Can you work these out from the model? Positions are in its coordinate system, mm. A direction names the side the tool comes from. Coordinates: 2 decimals unless noted, no trailing zeros. Order: outer loops, then holes, each group sorted by start corner. A loop starts at its lowest first (then second) coordinate and runs counter-clockwise, first axis right, second up. Notation, with made-up numbers: (-4.5, 19) -> (0.5, 19) arc R6 ccw to (0.5, 29) -> close; hole circle Ø5 at (45.25, -4.75). An arc over 180 degrees is marked (long way). Answer in a Markdown table with one row per item. Add a question column.
1. Imagine slicing it at C-C on x = 0. State how many separate pieces and enclosed holes the cut face has, plus the area to 3 significant figures.
2. On a 3-axis mill with a long thin cutter (end or side, diameter ignored), from which of +Z, -Z, +X, -X, +Y, -Y can I reach the whole of each face in a straight line? I mean faces 5 (the face through (52.997, 6.958, -0.535)), 6 (the face through (34, 20, 15)), 7 (the face through (15, 2, 22)). Say none if no direction works.
3. Imagine slicing it at B-B on y = 6.25. Write out the boundary of the cut face in (x, z), plus the area to 3 significant figures.
4. If I drill on line 1 along Y through (x, z) = (-16, -44); line 2 along Z through (x, y) = (12, 19); line 3 along X through (y, z) = (9.5, -24), over which ranges is the centre line in solid material (lowest first)? Write a range as [from, to].
5. Imagine slicing it at A-A on y = 19.75. Write out the boundary of the cut face in (x, z).
6. Will these pins go through, and if not, where does the flat tip stop? pin 1 (5 mm diameter, centred on x = 39, y = 11, fed in from +Z); pin 2 (3 mm diameter, centred on x = 1.5, y = 2, fed in from +Z); pin 3 (5 mm diameter, centred on y = 4, z = 29, fed in from +X); pin 4 (1.6 mm diameter, centred on x = 35, y = 20, fed in from +Z).
7. We'd pull the mould along Z, two halves only. Please class faces 1 (the face through (0, 2, 17)), 2 (the face through (-0.642, 6.958, 38.995)), 3 (the face through (41, 9, -35)), 4 (the face through (-15, 2, -22)): pulls with the +Z half, pulls with the -Z half, needs draft (parallel to the pull), parting line crosses it, or undercut.
from build123d import *
from build123d.topology import SkipClean

# Parameters (mm, degrees)
SKETCH_1_R          = 55.00000000000001
EXTRUDE_1_DEPTH     = 4
EXTRUDE_2_DEPTH     = 10
SKETCH_3_R          = 1.499999999999999
SKETCH_3_R_2        = 1.500000000000004
CUT_EXTRUDE_1_DEPTH = 6
FILLET_1_R          = 1
EXTRUDE_3_DEPTH     = 10
SKETCH_5_R          = 55.00000000000001
SKETCH_5_R_2        = 36
EXTRUDE_4_DEPTH     = 4
SKETCH_6_R          = 55.00000000000001
SKETCH_6_R_2        = 53
EXTRUDE_5_DEPTH     = 5
CUT_EXTRUDE_START   = -4
CUT_EXTRUDE_2_DEPTH = 4
FILLET_2_R          = 4
CUT_EXTRUDE_3_DEPTH = 10
FILLET_3_R          = 3


with BuildPart() as part:
    # 草图1 → 凸台-拉伸1 (new body)
    with BuildSketch(Plane(origin=(0, 0, 0), x_dir=(1, 0, 0), z_dir=(0, 1, 0))):
        with Locations(Location((0, 0, 0), (0, 0, 270))):
            Circle(SKETCH_1_R)
    extrude(amount=EXTRUDE_1_DEPTH)

    # 草图2 → 凸台-拉伸2 (add)
    with BuildSketch(Plane(origin=(0, 4, 0), x_dir=(1, 0, 0), z_dir=(0, 1, 0))):
        with BuildLine():
            Line((-39.799497484264805, 35), (-42.42640687119287, 35))
            ThreePointArc((-42.42640687119286, 35.000000000000014), (-55.000000000000014, 6.74e-15), (-42.42640687119287, -35))
            Line((-42.42640687119284, -35), (-39.799497484264776, -35))
            ThreePointArc((-39.79949748426479, -35.00000000000001), (-53, 6.49e-15), (-39.799497484264805, 35))
        make_face()
        with BuildLine():
            ThreePointArc((55.000000000000014, 0), (51.76124215045274, 18.59499424689872), (42.426406871192874, 35))
            Line((42.42640687119287, 35), (39.799497484264805, 35))
            ThreePointArc((39.799497484264805, 35), (49.59018736940825, 18.703296946447246), (53, 0))
            ThreePointArc((53, -1.298e-14), (49.590187369408234, -18.703296946447267), (39.799497484264776, -35.00000000000002))
            Line((39.799497484264776, -35), (42.42640687119284, -35))
            ThreePointArc((42.42640687119285, -35.00000000000002), (51.76124215045274, -18.594994246898718), (55.000000000000014, -1.347e-14))
        make_face()
    extrude(amount=EXTRUDE_2_DEPTH)

    # 草图3 → 切除-拉伸1 (cut)
    with BuildSketch(Plane.XZ):
        with Locations(Location((14.85, 5, 0), (0, 0, 270))):
            Circle(SKETCH_3_R)
        with Locations(Location((14.85, -5, 0), (0, 0, 90))):
            Circle(SKETCH_3_R)
        with Locations(Location((-34.65, 5, 0), (0, 0, 270))):
            Circle(SKETCH_3_R_2)
        with Locations(Location((-34.65, -5, 0), (0, 0, 90))):
            Circle(SKETCH_3_R_2)
        Polygon((-31.4, -10.999999999999996), (11.599999999999998, -10.999999999999996), (11.599999999999994, 11.000000000000004), (-31.4, 11.000000000000004), align=None)
    extrude(amount=-CUT_EXTRUDE_1_DEPTH, mode=Mode.SUBTRACT)

    # 圆角1
    fillet_1_edges = [part.edges().sort_by_distance(p)[0] for p in [
        (11.599999999999994, 2, 11.000000000000004),
        (11.599999999999998, 2, -10.999999999999996),
        (-31.4, 2, -10.999999999999996),
        (-31.4, 2, 11.000000000000004),
    ]]
    fillet(fillet_1_edges, radius=FILLET_1_R)

    # 草图4 → 凸台-拉伸3 (add)
    with BuildSketch(Plane(origin=(0, 4, 0), x_dir=(1, 0, 0), z_dir=(0, 1, 0))):
        with BuildLine():
            ThreePointArc((-32.72613634390714, 14.999999999999996), (-5.79e-15, 36), (32.72613634390714, 14.999999999999996))
            Line((32.72613634390714, 14.999999999999996), (36.00000000000001, 14.999999999999996))
            ThreePointArc((36, 14.999999999999995), (2.39e-15, 39), (-36, 14.999999999999998))
            Line((-36.00000000000001, 14.999999999999996), (-32.72613634390714, 14.999999999999996))
        make_face()
        with BuildLine():
            Line((36, -15.000000000000014), (32.726136343907136, -15.000000000000014))
            ThreePointArc((32.72613634390713, -15.000000000000028), (-6.61e-15, -36), (-32.726136343907136, -15.000000000000016))
            Line((-32.726136343907136, -15.000000000000014), (-36, -15.000000000000014))
            ThreePointArc((-36, -15.000000000000005), (-7.16e-15, -39), (35.99999999999999, -15.000000000000018))
        make_face()
    extrude(amount=EXTRUDE_3_DEPTH)

    # 草图5 → 凸台-拉伸4 (add)
    with SkipClean():  # the faces are left unmerged after this step: merging them gives an invalid solid
        with BuildSketch(Plane(origin=(0, 14, 0), x_dir=(1, 0, 0), z_dir=(0, 1, 0))):
            with Locations(Location((0, 0, 0), (0, 0, 270))):
                Circle(SKETCH_5_R)
            with Locations(Location((0, 0, 0), (0, 0, 155.375681648))):
                Circle(SKETCH_5_R_2, mode=Mode.SUBTRACT)
        extrude(amount=EXTRUDE_4_DEPTH)

    # 草图6 → 凸台-拉伸5 (add)
    # profile 1 of 3: a face of its own
    with SkipClean():  # the faces are left unmerged after this step: merging them gives an invalid solid
        with BuildSketch(Plane(origin=(0, 18.000000000000004, 0), x_dir=(1, 0, 0), z_dir=(0, 1, 0))):
            with Locations(Location((0, 0, 0), (0, 0, 270))):
                Circle(SKETCH_6_R)
            with Locations(Location((0, 0, 0), (0, 0, 270))):
                Circle(SKETCH_6_R_2, mode=Mode.SUBTRACT)
        # profile 2 of 3: a face of its own
        with BuildSketch(Plane(origin=(0, 18.000000000000004, 0), x_dir=(1, 0, 0), z_dir=(0, 1, 0))):
            with BuildLine():
                Line((-36.00000000000001, 14.999999999999996), (-32.72613634390714, 14.999999999999996))
                ThreePointArc((-32.72613634390714, 14.999999999999996), (-5.79e-15, 36), (32.72613634390714, 14.999999999999996))
                Line((32.72613634390714, 14.999999999999996), (36.00000000000001, 14.999999999999996))
                ThreePointArc((36, 14.999999999999995), (2.39e-15, 39), (-36, 14.999999999999998))
            make_face()
        # profile 3 of 3: a face of its own
        with BuildSketch(Plane(origin=(0, 18.000000000000004, 0), x_dir=(1, 0, 0), z_dir=(0, 1, 0))):
            with BuildLine():
                Line((36, -15.000000000000014), (32.726136343907136, -15.000000000000014))
                ThreePointArc((32.72613634390713, -15.000000000000028), (-6.61e-15, -36), (-32.726136343907136, -15.000000000000016))
                Line((-32.726136343907136, -15.000000000000014), (-36, -15.000000000000014))
                ThreePointArc((-36, -15.000000000000005), (-7.16e-15, -39), (35.99999999999999, -15.000000000000018))
            make_face()
        extrude(amount=EXTRUDE_5_DEPTH)

    # 草图7 → 切除-拉伸2 (cut)
    with BuildSketch(Plane(origin=(0, 18.000000000000004, 0), x_dir=(1, 0, 0), z_dir=(0, 1, 0)).offset(CUT_EXTRUDE_START)):
        with BuildLine():
            ThreePointArc((-36, -15.000000000000014), (-39.00000000000001, -4.78e-15), (-36.00000000000001, 14.999999999999996))
            Line((-36.00000000000001, 14.999999999999996), (-32.72613634390714, 14.999999999999996))
            ThreePointArc((-32.72613634390714, 14.999999999999996), (-36, -2.04e-14), (-32.726136343907136, -15.000000000000014))
            Line((-32.726136343907136, -15.000000000000014), (-36, -15.000000000000014))
        make_face()
    extrude(amount=CUT_EXTRUDE_2_DEPTH, mode=Mode.SUBTRACT)

    # 圆角2
    # the kernel refuses this fillet: 4 mm, written as the material it adds along each edge
    with BuildSketch(Plane(origin=(-3.55e-15, 14, -5.33e-15), x_dir=(0.9904724769404064, 0, -0.13771082899879708), z_dir=(0.13771082899879708, 0, 0.9904724769404064))) as fillet_2_piece_1_section:
        with BuildLine():
            CenterArc((39 + FILLET_2_R, -FILLET_2_R), FILLET_2_R, 90, 90)
            Line((39 + FILLET_2_R, 0), (39, 0))
            Line((39, 0), (38.99999999999999, -FILLET_2_R))
        make_face()
    fillet_2_piece_1 = revolve(axis=Axis((-3.55e-15, 14, -5.33e-15), (0, 1, 0)), revolution_arc=164.16919327842925, mode=Mode.PRIVATE)
    fillet_2_piece_1 = split(fillet_2_piece_1, bisect_by=Plane(origin=(0, 12.877029486971129, -14.999999999999996), z_dir=(0, 0, -1)), keep=Keep.TOP, mode=Mode.PRIVATE)
    add(fillet_2_piece_1)
    with BuildSketch(Plane(origin=(3.55e-15, 14, -8.88e-15), x_dir=(-0.9904724769404064, 0, 0.13771082899879786), z_dir=(-0.13771082899879786, 0, -0.9904724769404064))) as fillet_2_piece_2_section:
        with BuildLine():
            CenterArc((38.99999999999986 + FILLET_2_R, -FILLET_2_R), FILLET_2_R, 90, 90)
            Line((38.99999999999986, -FILLET_2_R), (38.99999999999986, 0))
            Line((38.99999999999986, 0), (38.99999999999986 + FILLET_2_R, 0))
        make_face()
    fillet_2_piece_2 = revolve(axis=Axis((3.55e-15, 14, -8.88e-15), (0, 1, 0)), revolution_arc=164.16919327842916, mode=Mode.PRIVATE)
    fillet_2_piece_2 = split(fillet_2_piece_2, bisect_by=Plane(origin=(-7.11e-15, 12.877029483112029, 15.000000000000014), z_dir=(0, 0, 1)), keep=Keep.TOP, mode=Mode.PRIVATE)
    add(fillet_2_piece_2)
    with BuildSketch(Plane(origin=(-4.263e-14, 14, -1.865e-14), x_dir=(0.6136949496452997, 0, 0.7895432279361612), z_dir=(-0.7895432279361612, 0, 0.6136949496452997))) as fillet_2_piece_3_section:
        with BuildLine():
            CenterArc((53.00000000000012 - FILLET_2_R, -FILLET_2_R), FILLET_2_R, 0, 90)
            Line((53.00000000000012, -FILLET_2_R), (53.00000000000012, 0))
            Line((53.00000000000012, 0), (53.00000000000012 - FILLET_2_R, 0))
        make_face()
    fillet_2_piece_3 = revolve(axis=Axis((-4.263e-14, 14, -1.865e-14), (0, 1, 0)), revolution_arc=104.28569181085327, mode=Mode.PRIVATE)
    fillet_2_piece_3 = split(fillet_2_piece_3, bisect_by=Plane(origin=(51.873764077248, 12.873764077247905, -35), z_dir=(0, 0, 1)), keep=Keep.TOP, mode=Mode.PRIVATE)
    fillet_2_piece_3 = split(fillet_2_piece_3, bisect_by=Plane(origin=(51.873764077248, 12.873764077247905, 35), z_dir=(0, 0, -1)), keep=Keep.TOP, mode=Mode.PRIVATE)
    add(fillet_2_piece_3)
    with BuildSketch(Plane(origin=(-1.421e-14, 14, -7.11e-15), x_dir=(-0.6136949496452995, 0, 0.7895432279361616), z_dir=(0.7895432279361616, 0, 0.6136949496452995))) as fillet_2_piece_4_section:
        with BuildLine():
            CenterArc((53.00000000000001 - FILLET_2_R, FILLET_2_R), FILLET_2_R, 270, 90)
            Line((53.00000000000001, FILLET_2_R), (53.00000000000001, 0))
            Line((53.00000000000001, 0), (53.00000000000001 - FILLET_2_R, 0))
        make_face()
    fillet_2_piece_4 = revolve(axis=Axis((-1.421e-14, 14, -7.11e-15), (0, -1, 0)), revolution_arc=104.28569181085335, mode=Mode.PRIVATE)
    fillet_2_piece_4 = split(fillet_2_piece_4, bisect_by=Plane(origin=(-51.87376407724794, 12.873764077247902, -35), z_dir=(0, 0, 1)), keep=Keep.TOP, mode=Mode.PRIVATE)
    fillet_2_piece_4 = split(fillet_2_piece_4, bisect_by=Plane(origin=(-51.87376407724794, 12.873764077247902, 35), z_dir=(0, 0, -1)), keep=Keep.TOP, mode=Mode.PRIVATE)
    add(fillet_2_piece_4)

    # 草图8 → 切除-拉伸3 (cut)
    with BuildSketch(Plane(origin=(0, 4, 0), x_dir=(1, 0, 0), z_dir=(0, 1, 0))):
        Polygon((-14.999999999999998, -27), (15.000000000000002, -27), (15.000000000000004, -16.999999999999996), (-14.999999999999996, -16.999999999999996), align=None)
        Polygon((-14.999999999999996, 16.999999999999996), (15.000000000000004, 16.999999999999996), (15.000000000000002, 27), (-14.999999999999998, 27), align=None)
    extrude(amount=-CUT_EXTRUDE_3_DEPTH, mode=Mode.SUBTRACT)

    # 圆角3
    fillet_3_edges = [part.edges().sort_by_distance(p)[0] for p in [
        (15.000000000000002, 2, -27),
        (15.000000000000004, 2, -16.999999999999996),
        (-14.999999999999996, 2, -16.999999999999996),
        (-14.999999999999998, 2, -27),
        (-14.999999999999998, 2, 27),
        (-14.999999999999996, 2, 16.999999999999996),
        (15.000000000000004, 2, 16.999999999999996),
        (15.000000000000002, 2, 27),
    ]]
    fillet(fillet_3_edges, radius=FILLET_3_R)


solid = part.part
Answers follow:
| question | item | result |
|---|---|---|
| 1 | separate pieces | 4 |
| 1 | enclosed holes | 0 |
| 1 | area | 541 mm² |
| 2 | face 5 | none |
| 2 | face 6 | +Y |
| 2 | face 7 | +Y, -Y |
| 3 | outline | (-42.43, -35) -> (-39.8, -35) arc R53 cw to (-39.8, 35) -> (-42.43, 35) arc R55 ccw to start; (-36, -15) arc R39 ccw to (36, -15) -> (32.73, -15) arc R36 cw to (-32.73, -15) -> close; (-36, 15) -> (-32.73, 15) arc R36 cw to (32.73, 15) -> (36, 15) arc R39 ccw to start; (39.8, -35) -> (42.43, -35) arc R55 ccw to (42.43, 35) -> (39.8, 35) arc R53 cw to start |
| 3 | area | 826 mm² |
| 4 | line 1 | y = [0, 4], [14, 18] |
| 4 | line 2 | z = [-53.67, -51.62], [-37.11, -33.94], [33.94, 37.11], [51.62, 53.67] |
| 4 | line 3 | x = [-49.49, -47.25], [-30.74, -26.83], [26.83, 30.74], [47.25, 49.49] |
| 5 | outline | circle Ø110 at (0, 0); (-36, -15) arc R39 ccw to (36, -15) -> (32.73, -15) arc R36 cw to (-32.73, -15) -> close; (-36, 15) -> (-32.73, 15) arc R36 cw to (32.73, 15) -> (36, 15) arc R39 ccw to start; hole circle Ø106 at (0, 0) |
| 6 | pin 1 | stops at z = 35 |
| 6 | pin 2 | stops at z = 55 |
| 6 | pin 3 | stops at x = 48.19 |
| 6 | pin 4 | stops at z = 43.07 |
| 7 | face 1 | undercut |
| 7 | face 2 | pulls with the +Z half |
| 7 | face 3 | pulls with the -Z half |
| 7 | face 4 | undercut |
